Model file for the job. Use its own axes, mm. A direction names the side the tool comes from. Round coordinates to 2 decimals unless told otherwise and drop trailing zeros. Order: outer loops, then holes, each group sorted by start corner. A loop starts at its lowest first (then second) coordinate and runs counter-clockwise, first axis right, second up. Notation, with made-up numbers: (-29.5, 18) - (-9.5, 18) arc R7 ccw to (-9.5, 30) - close; hole circle Ø11 at (49, -23). An arc over 180 degrees is marked (long way). Write item = value, one per line.
```python
from build123d import *

# Parameters (mm, degrees)
F2_R     = 19.8501
F3_DEPTH = 5.55625
F5_DEPTH = 254


with BuildPart() as f1:
    # F0 (on Front) → F1 (revolve)
    with BuildSketch(Plane.XZ):
        Polygon((0.150096, 0), (0, 0), (-3.29596, 0), (-7.690672, 12.7), (-10.826997, 12.7), (-10.826997, 9.985023), (-8.93062, 9.985023), (-6.797195, 0), (-6.797195, -4.826381), (-6.797195, -16.51), (6.833015, -16.51), (6.833015, 12.7), (4.501328, 12.7), align=None)
    revolve(axis=Axis((0.01791, 0, -16.51), (1, 0, 0)))

    # F2 (on face) → F3 (join)
    with BuildSketch(Plane.YZ.offset(6.833015)):
        with Locations((0, -16.51)):
            Circle(F2_R)
    extrude(amount=F3_DEPTH)

    # F4 (on face) → F5 (cut)
    with BuildSketch(Plane.YZ.offset(12.389265)):
        with BuildLine():
            Line((-2.39395, -4.851507), (-2.39395, -7.264507))
            ThreePointArc((-2.39395, -7.264507), (0, -26.0604), (2.39395, -7.264507))
            Line((2.39395, -7.264507), (2.39395, -4.851507))
            Line((2.39395, -4.851507), (0, -4.851507))
            Line((0, -4.851507), (-2.39395, -4.851507))
        make_face()
    extrude(amount=-F5_DEPTH, mode=Mode.SUBTRACT)


solid = f1.part
```
1) Mould opens along Y. For faces 6 (the face through (6.833, 19, -23)), 7 (the face through (3, 0, -4.852)), 8 (the face through (-3.571, -5.198, -0.005)) say: +Y half, -Y half, draft (parallel to the pull), parting line (faces both ways), or undercut.
Conclusion:
face_6 = draft
face_7 = undercut
face_8 = parting line
2) Flat gauge pins, fed straight in: pin 1 Ø1.5 at (y, z) = (10.5, -36.5) entering from +X; pin 2 Ø12 at (x, y) = (2, 6.5) entering from -Z; pin 3 Ø3 at (y, z) = (10, -30) entering from -X. Where does each tip first touch, or does it go through?
Conclusion:
pin_1 = 6.83
pin_2 = -45.7
pin_3 = -7.18
3) Wall check: line 1 along Y through (x, z) = (-10.15, -16.51); line 2 along Z through (x, y) = (-9.25, 0); line 3 along Z through (x, y) = (-1.5, -0.5). Give the ranges that are in metal, low to high.
Conclusion:
line_1 = -29.21 to -26.5, 26.5 to 29.21
line_2 = -45.72 to -43.01, 9.99 to 12.7
line_3 = -33.01 to -26.05, -4.85 to -0.01
4) Cut at A-A (x = 9.75). Write the cut outline in (y, z), and give its area (3 significant figures).
Conclusion:
outline = circle Ø39.7 at (0, -16.51); hole (-2.39, -7.26) arc R9.55 ccw (long way) to (2.39, -7.26) - (2.39, -4.85) - (-2.39, -4.85) - close
area = 941 mm^2
5) 3-axis set-ups, long thin cutter, end or side, ignore diameter. For faces 1 (the face through (-10.827, 26, -10)), 2 (the face through (9.572, 18.933, -10.548)), 3 (the face through (3, -2.394, -6)), 4 (the face through (-6.797, 7, -9)), 5 (the face through (-1.597, -4.959, -0.762)): which of +Z, -Z, +X, -X, +Y, -Y reach the whole face in a straight line?
Conclusion:
face_1 = +Z, -Z, -X, +Y, -Y
face_2 = +X
face_3 = +X, -X
face_4 = -X
face_5 = none
6) Cut at C-C (z = -16.51). Write the cut outline in (x, y).
Conclusion:
outline = (-10.83, -29.21) - (-7.69, -29.21) - (-3.3, -16.51) - (0.15, -16.51) - (4.5, -29.21) - (6.83, -29.21) - (6.83, -19.85) - (12.39, -19.85) - (12.39, -9.55) - (-6.8, -9.55) - (-6.8, -16.51) - (-8.93, -26.5) - (-10.83, -26.5) - close; (-10.83, 26.5) - (-8.93, 26.5) - (-6.8, 16.51) - (-6.8, 9.55) - (12.39, 9.55) - (12.39, 19.85) - (6.83, 19.85) - (6.83, 29.21) - (4.5, 29.21) - (0.15, 16.51) - (-3.3, 16.51) - (-7.69, 29.21) - (-10.83, 29.21) - close
7) Cut at B-B (y = 0). Write the cut outline in (x, z), and give its area (3 significant figures).
Conclusion:
outline = (-10.83, -45.72) - (-7.69, -45.72) - (-3.3, -33.02) - (0.15, -33.02) - (4.5, -45.72) - (6.83, -45.72) - (6.83, -36.36) - (12.39, -36.36) - (12.39, -26.06) - (-6.8, -26.06) - (-6.8, -33.02) - (-8.93, -43.01) - (-10.83, -43.01) - close; (-10.83, 9.99) - (-8.93, 9.99) - (-6.8, 0) - (-6.8, -4.85) - (12.39, -4.85) - (12.39, 3.34) - (6.83, 3.34) - (6.83, 12.7) - (4.5, 12.7) - (0.15, 0) - (-3.3, 0) - (-7.69, 12.7) - (-10.83, 12.7) - close
area = 455 mm^2
8) Cut at D-D (x = -2.5). Write the cut outline in (y, z), and give its area (3 significant figures).
Conclusion:
outline = circle Ø33.02 at (0, -16.51); hole (-2.39, -7.26) arc R9.55 ccw (long way) to (2.39, -7.26) - (2.39, -4.85) - (-2.39, -4.85) - close
area = 559 mm^2
